```python
from build123d import *

# Parameters (mm, degrees)
BOSS_EXTRUDE1_DEPTH = 5.08
SKETCH2_W           = 6.35
SKETCH2_H           = 5.08
CUT_EXTRUDE1_DEPTH  = 6.08
LPATTERN1_COUNT     = 5
LPATTERN1_PITCH     = 19.05


with BuildPart() as part:
    # Sketch1 → Boss-Extrude1 (new body)
    with BuildSketch(Plane(origin=(0, 0, 0), x_dir=(1, 0, 0), z_dir=(0, 1, 0))):
        Polygon((0, 12.7), (0, 19.05), (124.46, 19.05), (124.46, 12.7), (119.38, 12.7), (119.38, 6.35), (124.46, 6.35), (124.46, 0), (0, 0), (0, 6.35), (5.08, 6.35), (5.08, 12.7), align=None)
    extrude(amount=BOSS_EXTRUDE1_DEPTH)

    # Sketch2 → Cut-Extrude1 (cut, through all)
    with BuildSketch(Plane(origin=(0, 5.08, 0), x_dir=(1, 0, 0), z_dir=(0, 1, 0))):
        with Locations((24.13, 9.525)):
            Rectangle(SKETCH2_W, SKETCH2_H)
    cut_extrude1 = extrude(amount=-CUT_EXTRUDE1_DEPTH, mode=Mode.SUBTRACT)

    # LPattern1: Cut-Extrude1 ×5
    with Locations(*[(i * LPATTERN1_PITCH, 0, 0) for i in range(1, LPATTERN1_COUNT)]):
        add(cut_extrude1, mode=Mode.SUBTRACT)


solid = part.part
```
Can you work these out from the model? Positions are in its coordinate system, mm. A direction names the side the tool comes from. Coordinates: 2 decimals unless noted, no trailing zeros. Write each loop counter-clockwise with the first axis right and the second up, starting at its lowest first coordinate (ties: lowest second). Pieces come first, ordered by that corner, then holes. Notation, with made-up numbers: (36, 46) - (58, 46) arc R23 ccw to (58, 61) - close; hole circle Ø10 at (71, 57.25). An arc over 180 degrees is marked (long way). Return JSON: item names as keys, results as strings.
Q1. I'm going to push flat-ended pins straight in: pin 1 Ø1.5 at (y, z) = (2, -9) entering from +X; pin 2 Ø1.5 at (x, z) = (18.5, -3) entering from -Y; pin 3 Ø2.5 at (y, z) = (3, -8.5) entering from -X. Where does each tip first touch, or does it pass through?
Computed values:
{"pin 1": "stops at x = 119.38", "pin 2": "stops at y = 0", "pin 3": "stops at x = 5.08"}
Q2. If we section it at B-B (y = 0.85): Count the separate pieces of the cut face and the enclosed holes in it, then the cut area to 3 significant figures.
Computed values:
{"separate pieces": "1", "enclosed holes": "5", "area": "2,150 mm2"}
Q3. Thinking about a two-plate mould opening in X: for faces 4 (the flat face through (0, 3, -3)), 5 (the flat face through (81, 3, -12.065)), 6 (the flat face through (124.46, 3, -16)), which applies, +X half, -X half, draft (parallel to the pull), parting line (faces both ways), or undercut?
Computed values:
{"face 4": "-X half", "face 5": "undercut", "face 6": "+X half"}
Q4. If we section it at A-A (z = -9): Please give me the cut outline in (x, y) (3 decimals).
Computed values:
{"outline": "(5.08, 0) - (20.955, 0) - (20.955, 5.08) - (5.08, 5.08) - close; (27.305, 0) - (40.005, 0) - (40.005, 5.08) - (27.305, 5.08) - close; (46.355, 0) - (59.055, 0) - (59.055, 5.08) - (46.355, 5.08) - close; (65.405, 0) - (78.105, 0) - (78.105, 5.08) - (65.405, 5.08) - close; (84.455, 0) - (97.155, 0) - (97.155, 5.08) - (84.455, 5.08) - close; (103.505, 0) - (119.38, 0) - (119.38, 5.08) - (103.505, 5.08) - close"}
Q5. On a 3-axis mill with a long thin cutter (end or side, diameter ignored), from which of +Z, -Z, +X, -X, +Y, -Y can I reach the whole of each face in a straight line? I mean faces 1 (the flat face through (43, 3, -12.065)), 2 (the flat face through (122, 3, -12.7)), 3 (the flat face through (3, 3, -6.35)). Say none if no direction works.
Computed values:
{"face 1": "+Y, -Y", "face 2": "+X, +Y, -Y", "face 3": "-X, +Y, -Y"}
Q6. Please list where these lines run through material, in increasing order: L1, parallel to X at y = 3.9, z = -11.5 (3 decimals); L2, parallel to Z at x = 65, y = 3.3 (3 decimals); L3, parallel to X at y = 2.75, z = -12.25. Write a range as from..to.
Computed values:
{"L1": "x = 5.08..20.955, 27.305..40.005, 46.355..59.055, 65.405..78.105, 84.455..97.155, 103.505..119.38", "L2": "z = -19.05..-12.065, -6.985..0", "L3": "x = 5.08..119.38"}
